```python
from build123d import *

# Parameters (mm, degrees)
F0_W          = 1320.8
F0_H          = 304.8
F1_DEPTH      = 19.05
F2_R          = 139.7
F3_DEPTH      = 76.2
F3_DEPTH_BACK = 76.2


with BuildPart() as f1:
    # F0 (on Right) → F1 (new body)
    with BuildSketch(Plane.YZ):
        with Locations((660.4, 152.4)):
            Rectangle(F0_W, F0_H)
    extrude(amount=F1_DEPTH)

    # F2 (on face) → F3 (join, two sides)
    with BuildSketch(Plane.YZ.offset(19.05)) as f3_sk:
        with Locations((254, 152.4)):
            Circle(F2_R)
    extrude(amount=F3_DEPTH)
    extrude(f3_sk.sketch, amount=-F3_DEPTH_BACK)


solid = f1.part
```
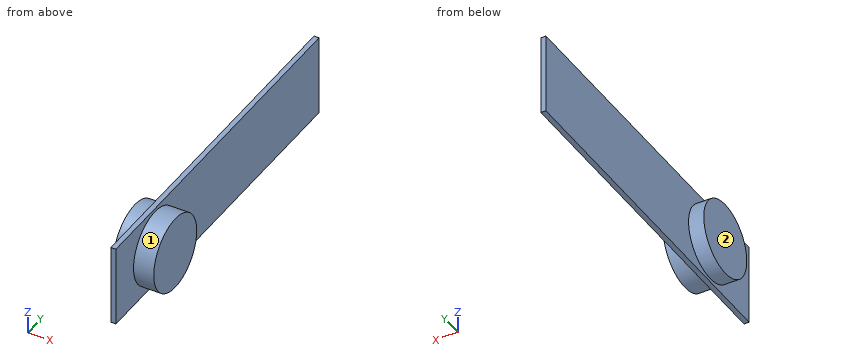
The listing builds one solid part. Answer for the finished solid, in the listing's coordinates (mm). Face numbers are marked on the shaded views. A direction names the side the tool comes from. Round coordinates to 2 decimals unless told otherwise and drop trailing zeros. Order: outer loops, then holes, each group sorted by start corner. A loop starts at its lowest first (then second) coordinate and runs counter-clockwise, first axis right, second up. Notation, with made-up numbers: (-35, 37.25) - (-21, 37.25) arc R21 cw to (-21, 52.25) - close; hole circle Ø2 at (35.5, 72.5). An arc over 180 degrees is marked (long way). Put each result on its own line as item: value. Start each with the question number.
(1) Straight lines are drawn through the part: probe 1 along X at (y, z) = (925, 121); probe 2 along Y at (x, z) = (72.5, 151); probe 3 along Z at (x, y) = (59, 349). For each, find the intervals that lie inside material, in ascending order. Write a range as from..to.
(2) Find section C-C (x = 71.5). Give the vertices of the cut face in (y, z).
(3) Find section B-B (z = 84). Give the vertices of the cut face in (x, y), plus the area to 3 significant figures.
(4) Find section D-D (y = 1174). Give the vertices of the cut face in (x, z).
(5) Given P1, Ø8, axis at y = 497, z = 84.5, coming from the +X side; P2, Ø12, axis at x = 73.5, z = 272.5, coming from the +Y side; P3, Ø1.5, axis at y = 402.5, z = 75, coming from the -X side, each flat-ended and moving along its own axis, determine where each tip first touches the part or whether it passes through.
(6) For the marked faces 1 and 2, determine the directions among +Z, -Z, +X, -X, +Y, -Y from which every point of the face is accessible in a straight line to the end or side of a thin tool.
(7) Find section A-A (y = 254). Give the vertices of the cut face in (x, z), plus the area to 3 significant figures.
Reply:
1. probe 1: 0..19.05
1. probe 2: 114.31..393.69
1. probe 3: 49.97..254.83
2. outline: circle Ø279.4 at (254, 152.4)
3. outline: (-57.15, 132.19) - (0, 132.19) - (0, 0) - (19.05, 0) - (19.05, 132.19) - (95.25, 132.19) - (95.25, 375.81) - (19.05, 375.81) - (19.05, 1320.8) - (0, 1320.8) - (0, 375.81) - (-57.15, 375.81) - close
3. area: 57,600 mm^2
4. outline: (0, 0) - (19.05, 0) - (19.05, 304.8) - (0, 304.8) - close
5. P1: x = 19.05
5. P2: y = 334.61
5. P3: x = 0
6. face 1: +X
6. face 2: +Z, -Z, -X, +Y, -Y
7. outline: (-57.15, 12.7) - (0, 12.7) - (0, 0) - (19.05, 0) - (19.05, 12.7) - (95.25, 12.7) - (95.25, 292.1) - (19.05, 292.1) - (19.05, 304.8) - (0, 304.8) - (0, 292.1) - (-57.15, 292.1) - close
7. area: 43,100 mm^2
